Check sheet for the modelled part. Datum: model origin and axes. Units: mm. A direction names the side the tool comes from. Round coordinates to 2 decimals unless told otherwise and drop trailing zeros. Write each loop counter-clockwise with the first axis right and the second up, starting at its lowest first coordinate (ties: lowest second). Pieces come first, ordered by that corner, then holes.
Item 1: Release check for a two-part mould opening along Y. For faces 1 (the cylindrical face through (2.974, 1.648, -9.443)), 2 (the cylindrical face through (-6.98, -1.67, 7.09)), 3 (the flat face through (2, 23.9, 13)) record: pulls with the +Y half, pulls with the -Y half, needs draft (parallel to the pull), parting line crosses it, or undercut.
Item 2: Section check B-B, the plane x = 0. Record the cut outline in (y, z) (3 decimals).
Item 3: Set-up check for faces 4 (the cylindrical face through (-10.8, -1.4, 0.1)), 5 (the cylindrical face through (10.8, -1.4, -0.1)), 6 (the flat face through (7, 11.39, -10)), 7 (the cylindrical face through (10.316, 17.816, 7.91)): record each of +Z, -Z, +X, -X, +Y, -Y from which the full face is reachable in a straight line by a thin tool's end or side.
Item 4: Section check C-C, the plane y = 16. Record the cut outline in (x, z) (3 decimals).
Item 5: Depth check by flat-ended pin: pin 1 (6 mm diameter, centred on y = 14, z = 6, fed in from -X); pin 2 (6 mm diameter, centred on y = 20.5, z = 5, fed in from -X); pin 3 (1.5 mm diameter, centred on x = -9.5, z = -7, fed in from -Y). Enter the tip coordinate at first touch or a pass-through.
Item 6: Section check A-A, the plane y = -0.5. Record the cut outline in (x, z).
Item 7: Section check D-D, the plane y = 4.5. Record the cut outline in (x, z) (3 decimals), plus the area to 3 significant figures.
Item 8: Material ranges on line 1 along Y through (x, z) = (0.5, -0.25); line 2 along Y through (x, z) = (9, -5); line 3 along Z through (x, y) = (4, 21), recorded low to high.
from build123d import *

# Parameters (mm, degrees)
BOSS_EXTRUDE1_DEPTH       = 3.3
M22_CLEARANCE_HOLE1_D     = 26
M22_CLEARANCE_HOLE1_DEPTH = 12
CHAMFER1_SIZE             = 0.5
FILLET1_R                 = 0.5


with BuildPart() as part:
    # Sketch1 → Boss-Extrude1 (new body)
    with BuildSketch(Plane.XZ.offset(3.3)):
        with BuildLine():
            Line((-2.3, 10.052250945), (-2.3, 9.68052168))
            ThreePointArc((-2.3, 9.68052168), (-7.035712473, 7.035712473), (-9.68052168, 2.3))
            Line((-9.68052168, 2.3), (-9.897884029, 2.3))
            Line((-9.897884029, 2.3), (-10.64555554, 1.819930558))
            ThreePointArc((-10.64555554, 1.819930558), (-10.799781696, 0.06866818), (-10.667837189, -1.684413755))
            Line((-10.667837189, -1.684413755), (-10.052250945, -2.3))
            Line((-10.052250945, -2.3), (-9.68052168, -2.3))
            ThreePointArc((-9.68052168, -2.3), (-7.035712473, -7.035712473), (-2.3, -9.68052168))
            Line((-2.3, -9.68052168), (-2.3, -9.897884029))
            Line((-2.3, -9.897884029), (-1.819930558, -10.64555554))
            ThreePointArc((-1.819930558, -10.64555554), (-0.06866818, -10.799781696), (1.684413755, -10.667837189))
            Line((1.684413755, -10.667837189), (2.3, -10.052250945))
            Line((2.3, -10.052250945), (2.3, -9.68052168))
            ThreePointArc((2.3, -9.68052168), (7.035712473, -7.035712473), (9.68052168, -2.3))
            Line((9.68052168, -2.3), (9.897884029, -2.3))
            Line((9.897884029, -2.3), (10.64555554, -1.819930558))
            ThreePointArc((10.64555554, -1.819930558), (10.799781696, -0.06866818), (10.667837189, 1.684413755))
            Line((10.667837189, 1.684413755), (10.052250945, 2.3))
            Line((10.052250945, 2.3), (9.68052168, 2.3))
            ThreePointArc((9.68052168, 2.3), (7.035712473, 7.035712473), (2.3, 9.68052168))
            Line((2.3, 9.68052168), (2.3, 9.897884029))
            Line((2.3, 9.897884029), (1.819930558, 10.64555554))
            ThreePointArc((1.819930558, 10.64555554), (0.06866818, 10.799781696), (-1.684413755, 10.667837189))
            Line((-1.684413755, 10.667837189), (-2.3, 10.052250945))
        make_face()
    extrude(amount=-BOSS_EXTRUDE1_DEPTH)

    # Sketch2 → Revolve1 (revolve)
    with BuildSketch(Plane.XY, mode=Mode.PRIVATE) as revolve1_sk:
        Polygon((14.925, 23.9), (0, 23.9), (0, 0), (9.9, 0), (9.9, 3.25), (10.875, 3.25), (10.875, 10.05), (12, 10.05), (12, 11.39), (14.925, 11.39), align=None)
    revolve(revolve1_sk.sketch.rotate(Axis((0, 23.9, 0), (0, -1, 0)), 270), axis=Axis((0, 23.9, 0), (0, -1, 0)))

    # M22 Clearance Hole1
    with Locations(Plane(origin=(0, 23.9, 0), x_dir=(1, 0, 0), z_dir=(0, 1, 0))):
        with Locations((0, 0)):
            Hole(M22_CLEARANCE_HOLE1_D / 2, depth=M22_CLEARANCE_HOLE1_DEPTH)

    # Chamfer1
    chamfer1_edges = [part.edges().sort_by_distance(p)[0] for p in [
        (-10.799781696, -3.3, 0.06866818),
        (0.06866818, -3.3, 10.799781696),
        (-0.06866818, -3.3, -10.799781696),
        (10.799781696, -3.3, -0.06866818),
    ]]
    chamfer(chamfer1_edges, length=CHAMFER1_SIZE)

    # Fillet1
    fillet1_edges = [part.edges().sort_by_distance(p)[0] for p in [
        (0, 23.9, 14.925),
    ]]
    fillet(fillet1_edges, radius=FILLET1_R)


solid = part.part
Values found:
1. face 1: undercut
1. face 2: needs draft
1. face 3: pulls with the +Y half
2. outline: (-3.3, -10.3) - (-2.8, -10.8) - (0, -10.8) - (0, -9.9) - (3.25, -9.9) - (3.25, -10.875) - (10.05, -10.875) - (10.05, -12) - (11.39, -12) - (11.39, -14.925) - (23.4, -14.925) arc R0.5 ccw to (23.9, -14.425) - (23.9, -13) - (11.9, -13) - (11.9, 13) - (23.9, 13) - (23.9, 14.425) arc R0.5 ccw to (23.4, 14.925) - (11.39, 14.925) - (11.39, 12) - (10.05, 12) - (10.05, 10.875) - (3.25, 10.875) - (3.25, 9.9) - (0, 9.9) - (0, 10.8) - (-2.8, 10.8) - (-3.3, 10.3) - close
3. face 4: -X, -Y
3. face 5: +X, -Y
3. face 6: -Y
3. face 7: +Y
4. outline: circle Ø29.85 at (0, 0); hole circle Ø26 at (0, 0)
5. pin 1: stops at x = -14.62
5. pin 2: stops at x = -14.79
5. pin 3: stops at y = 10.05
6. outline: (-10.67, -1.68) - (-10.05, -2.3) - (-9.68, -2.3) arc R9.95 ccw to (-2.3, -9.68) - (-2.3, -9.9) - (-1.82, -10.65) arc R10.8 ccw to (1.68, -10.67) - (2.3, -10.05) - (2.3, -9.68) arc R9.95 ccw to (9.68, -2.3) - (9.9, -2.3) - (10.65, -1.82) arc R10.8 ccw to (10.67, 1.68) - (10.05, 2.3) - (9.68, 2.3) arc R9.95 ccw to (2.3, 9.68) - (2.3, 9.9) - (1.82, 10.65) arc R10.8 ccw to (-1.68, 10.67) - (-2.3, 10.05) - (-2.3, 9.68) arc R9.95 ccw to (-9.68, 2.3) - (-9.9, 2.3) - (-10.65, 1.82) arc R10.8 ccw to start
7. outline: circle Ø21.75 at (0, 0)
7. area: 372 mm2
8. line 1: y = -3.3 to 11.9
8. line 2: y = 3.25 to 11.9
8. line 3: z = -14.38 to -12.37, 12.37 to 14.38
